Verification items for the finished model (mm, model axes). A direction names the side the tool comes from. Coordinates: 2 decimals unless noted, no trailing zeros. Order: outer loops, then holes, each group sorted by start corner. A loop starts at its lowest first (then second) coordinate and runs counter-clockwise, first axis right, second up. Notation, with made-up numbers: (21.5, 86.25) -> (58.5, 86.25) arc R10 ccw to (58.5, 103.25) -> close; hole circle Ø11 at (-8.75, 12.5). An arc over 180 degrees is marked (long way). Answer as CSV lines item,"result".
```python
from build123d import *

# Parameters (mm, degrees)
EXTRUDE_1_DEPTH     = 150
CUT_EXTRUDE_START   = -140
CUT_EXTRUDE_1_DEPTH = 140
SKETCH_5_R          = 2.5
CUT_EXTRUDE_2_DEPTH = 302.021089881


with BuildPart() as part:
    # 草图1 → 凸台-拉伸1 (new body)
    with BuildSketch(Plane(origin=(0, 0, 0), x_dir=(1, 0, 0), z_dir=(0, 1, 0))):
        with BuildLine():
            Line((83.929371052, -4.001384199), (83.929371052, 45.998615801))
            ThreePointArc((83.929371052, 45.998615801), (78.929371052, 50.998615801), (73.929371052, 45.998615801))
            Line((73.929371052, 45.998615801), (73.929371052, -4.001384199))
            Line((73.929371052, -4.001384199), (73.929371052, -9.859248575))
            ThreePointArc((73.929371052, -9.859248575), (74.690575727, -13.686082899), (76.85830324, -16.930316387))
            Line((76.85830324, -16.930316387), (121.000438864, -61.072452011))
            ThreePointArc((121.000438864, -61.072452011), (123.168166377, -64.316685499), (123.929371052, -68.143519823))
            Line((123.929371052, -68.143519823), (123.929371052, -159.859248575))
            ThreePointArc((123.929371052, -159.859248575), (123.168166377, -163.686082899), (121.000438864, -166.930316387))
            Line((121.000438864, -166.930316387), (76.85830324, -211.072452011))
            ThreePointArc((76.85830324, -211.072452011), (74.690575727, -214.316685499), (73.929371052, -218.143519823))
            Line((73.929371052, -218.143519823), (73.929371052, -224.001384199))
            Line((73.929371052, -224.001384199), (131.000438864, -166.930316387))
            ThreePointArc((131.000438864, -166.930316387), (133.168166377, -163.686082899), (133.929371052, -159.859248575))
            Line((133.929371052, -159.859248575), (133.929371052, -68.143519823))
            ThreePointArc((133.929371052, -68.143519823), (133.168166377, -64.316685499), (131.000438864, -61.072452011))
            Line((131.000438864, -61.072452011), (86.85830324, -16.930316387))
            ThreePointArc((86.85830324, -16.930316387), (84.690575727, -13.686082899), (83.929371052, -9.859248575))
            Line((83.929371052, -9.859248575), (83.929371052, -4.001384199))
        make_face()
    extrude(amount=EXTRUDE_1_DEPTH)

    # 草图3 → 切除-拉伸1 (cut)
    with BuildSketch(Plane(origin=(0, 150, 0), x_dir=(1, 0, 0), z_dir=(0, 1, 0)).offset(CUT_EXTRUDE_START)):
        with BuildLine():
            Line((83.929371052, -9.859248575), (73.929371052, -9.859248575))
            Line((73.929371052, -9.859248575), (73.929371052, 45.998615801))
            ThreePointArc((73.929371052, 45.998615801), (78.929371052, 50.998615801), (83.929371052, 45.998615801))
            Line((83.929371052, 45.998615801), (83.929371052, -9.859248575))
        make_face()
    extrude(amount=CUT_EXTRUDE_1_DEPTH, mode=Mode.SUBTRACT)

    # 草图5 → 切除-拉伸2 (cut, through all)
    with BuildSketch(Plane.XZ):
        with Locations(Location((78.929371052, -45.998615801, 0), (0, 0, 270))):
            Circle(SKETCH_5_R)
        with Locations(Location((78.929371052, 4.001384199, 0), (0, 0, 270))):
            Circle(SKETCH_5_R)
    extrude(amount=-CUT_EXTRUDE_2_DEPTH, mode=Mode.SUBTRACT)


solid = part.part
```
Item 1: Section check A-A, the plane x = 109. Record the boundary of the cut face in (y, z).
Answer list:
outline,"(0, 39.07) -> (150, 39.07) -> (150, 49.07) -> (0, 49.07) -> close; (0, 178.93) -> (150, 178.93) -> (150, 188.93) -> (0, 188.93) -> close"
Item 2: Tool access check on faces 5 (the cylindrical face through (74.71, 73.95, 214.27)), 6 (the flat face through (79, 79, 9.859)), 7 (the cylindrical face through (76.49, 4.93, 4.54)). Record the directions out of +Z, -Z, +X, -X, +Y, -Y that give a thin tool (end or side, any length) a straight path to the whole face; none if there is none.
Answer list:
face 5,"-X, +Y, -Y"
face 6,"-Z, +X, -X, +Y"
face 7,"+Y, -Y"
Item 3: Release check for a two-part mould opening along Z. For faces 1 (the cylindrical face through (76.71, 4.93, -47.15)), 2 (the flat face through (79, 10, -21)), 3 (the cylindrical face through (79, 5, -51)), 4 (the flat face through (102.065, 73.95, 195.865)) record: +Z half, -Z half, draft (parallel to the pull), parting line (faces both ways), or undercut.
Answer list:
face 1,"undercut"
face 2,"draft"
face 3,"-Z half"
face 4,"+Z half"
Item 4: Section check C-C, the plane z = 135. Record the boundary of the cut face in (x, y), plus the area to 3 significant figures.
Answer list:
outline,"(123.93, 0) -> (133.93, 0) -> (133.93, 150) -> (123.93, 150) -> close"
area,"1,500 mm2"
Item 5: Section check D-D, the plane z = -26. Record the boundary of the cut face in (x, y).
Answer list:
outline,"(73.93, 0) -> (83.93, 0) -> (83.93, 10) -> (73.93, 10) -> close"
Item 6: Section check B-B, the plane y = 62.5. Record the boundary of the cut face in (x, z), plus the area to 3 significant figures.
Answer list:
outline,"(73.93, 9.86) -> (83.93, 9.86) arc R10 cw to (86.86, 16.93) -> (131, 61.07) arc R10 ccw to (133.93, 68.14) -> (133.93, 159.86) arc R10 ccw to (131, 166.93) -> (73.93, 224) -> (73.93, 218.14) arc R10 ccw to (76.86, 211.07) -> (121, 166.93) arc R10 cw to (123.93, 159.86) -> (123.93, 68.14) arc R10 cw to (121, 61.07) -> (76.86, 16.93) arc R10 ccw to start"
area,"2,090 mm2"
Item 7: Thickness scan on line 1 (X direction, y = 96, z = 106); line 2 (Z direction, x = 97, y = 134.5); line 3 (Z direction, x = 83, y = 61). Record the ranges inside material, lowest first.
Answer list:
line 1,"123.93 to 133.93"
line 2,"27.07 to 37.07, 190.93 to 200.93"
line 3,"9.86 to 23.07, 204.93 to 214.93"
Item 8: Depth check by flat-ended pin: pin 1 Ø3 at (y, z) = (7.5, -11.5) entering from +X; pin 2 Ø2 at (x, y) = (119, 87.5) entering from +Z; pin 3 Ø11 at (x, y) = (77, 53.5) entering from -Z. Enter the tip coordinate at first touch or a pass-through.
Answer list:
pin 1,"x = 83.93"
pin 2,"z = 179.93"
pin 3,"z = 9.86"
